Check sheet for the modelled part. Datum: model origin and axes. Units: mm. Face numbers are marked on the shaded views. A direction names the side the tool comes from. Give positions to 0.01 mm unless a question says otherwise; leave off trailing zeros. Order: outer loops, then holes, each group sorted by start corner. A loop starts at its lowest first (then second) coordinate and runs counter-clockwise, first axis right, second up.
Item 1: Access from +Z, -Z, +X, -X, +Y, -Y to the whole of each face (thin tool, end or side, straight path). Record for the marked faces 1 and 2.
Item 2: Gauge pin test, flat ends, axial feed: P1, Ø1.5, axis at x = -93, z = 33, coming from the -Y side; P2, Ø1.5, axis at y = 23, z = 33, coming from the +X side; P3, Ø25, axis at x = 22, y = -5, coming from the +Z side; P4, Ø3, axis at y = 16.5, z = 17.5, coming from the +X side. Record the tip position at first contact, or that the pin passes through.
Item 3: Sectioned sample at C-C on x = 61.5. Record the boundary of the cut face in (y, z), and give its area (3 significant figures).
Item 4: Release check for a two-part mould opening along Y. For the marked faces 3, 4 and 5 record: released by +Y, released by -Y, zero draft, split by the parting line, or undercut.
Item 5: Sectioned sample at B-B on y = -6. Record the boundary of the cut face in (x, z), and give its area (3 significant figures).
Item 6: Material ranges on line 1 along X through (y, z) = (-12.5, 21.5); line 2 along Y through (x, z) = (79.5, 27.5); line 3 along Z through (x, y) = (65.5, -17.5), recorded low to high.
Item 7: Sectioned sample at A-A on z = 10.5. Record the boundary of the cut face in (x, y), and give its area (3 significant figures).
from build123d import *

# Parameters (mm, degrees)
F0_R     = 2.5
F1_DEPTH = 32
F2_DEPTH = 35
F3_DEPTH = 4


with BuildPart() as f1:
    # F0 (on Top) → F1 (new body)
    with BuildSketch(Plane.XY):
        with BuildLine():
            Line((-95, 15), (-91, 15))
            ThreePointArc((-91, 15), (-89.242641, 19.242641), (-85, 21))
            Line((-85, 21), (-85, 25))
            ThreePointArc((-85, 25), (-92.071068, 22.071068), (-95, 15))
        make_face()
        with BuildLine():
            ThreePointArc((91, -15), (89.242641, -19.242641), (85, -21))
            Line((85, -21), (-85, -21))
            ThreePointArc((-85, -21), (-89.242641, -19.242641), (-91, -15))
            Line((-91, -15), (-91, 15))
            Line((-91, 15), (-95, 15))
            Line((-95, 15), (-95, -15))
            ThreePointArc((-95, -15), (-92.071068, -22.071068), (-85, -25))
            Line((-85, -25), (101, -25))
            ThreePointArc((101, -25), (108.071068, -22.071068), (111, -15))
            Line((111, -15), (111, 15))
            ThreePointArc((111, 15), (108.071068, 22.071068), (101, 25))
            Line((101, 25), (-85, 25))
            Line((-85, 25), (-85, 21))
            Line((-85, 21), (85, 21))
            ThreePointArc((85, 21), (89.242641, 19.242641), (91, 15))
            Line((91, 15), (91, -15))
        make_face()
        with Locations((101, 15)):
            Circle(F0_R, mode=Mode.SUBTRACT)
        with Locations((101, 15)):
            Circle(F0_R)
    extrude(amount=F1_DEPTH)

    # F0 (on Top) → F2 (join)
    with BuildSketch(Plane.XY):
        with BuildLine():
            Line((-95, 15), (-91, 15))
            ThreePointArc((-91, 15), (-89.242641, 19.242641), (-85, 21))
            Line((-85, 21), (-85, 25))
            ThreePointArc((-85, 25), (-92.071068, 22.071068), (-95, 15))
        make_face()
        with Locations((101, 15)):
            Circle(F0_R)
    extrude(amount=F2_DEPTH)

    # F0 (on Top) → F3 (join)
    with BuildSketch(Plane.XY):
        with BuildLine():
            Line((-85, -21), (85, -21))
            ThreePointArc((85, -21), (89.242641, -19.242641), (91, -15))
            Line((91, -15), (91, 15))
            ThreePointArc((91, 15), (89.242641, 19.242641), (85, 21))
            Line((85, 21), (-85, 21))
            ThreePointArc((-85, 21), (-89.242641, 19.242641), (-91, 15))
            Line((-91, 15), (-91, -15))
            ThreePointArc((-91, -15), (-89.242641, -19.242641), (-85, -21))
        make_face()
    extrude(amount=F3_DEPTH)


solid = f1.part
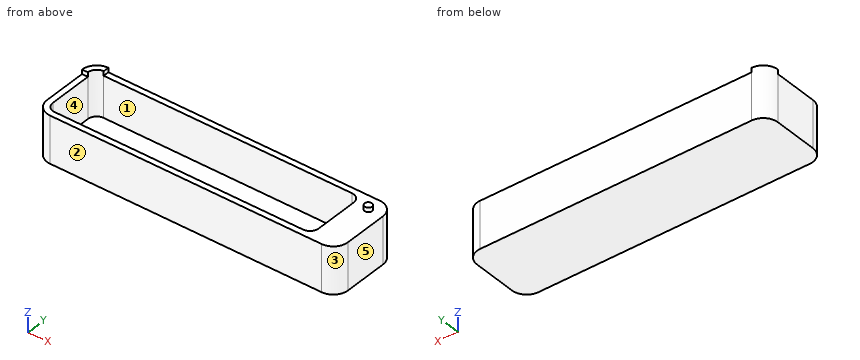
Report:
1. face 1: +Z
1. face 2: +Z, -Z, +X, -X, -Y
2. P1: stops at y = 15
2. P2: stops at x = -85
2. P3: stops at z = 4
2. P4: stops at x = 111
3. outline: (-25, 0) - (25, 0) - (25, 32) - (21, 32) - (21, 4) - (-21, 4) - (-21, 32) - (-25, 32) - close
3. area: 424 mm2
4. face 3: released by -Y
4. face 4: undercut
4. face 5: zero draft
5. outline: (-95, 0) - (111, 0) - (111, 32) - (91, 32) - (91, 4) - (-91, 4) - (-91, 32) - (-95, 32) - close
5. area: 1,500 mm2
6. line 1: x = -95 to -91, 91 to 111
6. line 2: y = -25 to -21, 21 to 25
6. line 3: z = 0 to 4
7. outline: (-95, -15) arc R10 ccw to (-85, -25) - (101, -25) arc R10 ccw to (111, -15) - (111, 15) arc R10 ccw to (101, 25) - (-85, 25) arc R10 ccw to (-95, 15) - close; hole (-91, -15) arc R6 ccw to (-85, -21) - (85, -21) arc R6 ccw to (91, -15) - (91, 15) arc R6 ccw to (85, 21) - (-85, 21) arc R6 ccw to (-91, 15) - close
7. area: 2,600 mm2
